Geometry check sheet. Reference: the model listing, model coordinates, mm. Give positions to 0.01 mm unless a question says otherwise; leave off trailing zeros. Write each loop counter-clockwise with the first axis right and the second up, starting at its lowest first coordinate (ties: lowest second). Pieces come first, ordered by that corner, then holes. Notation, with made-up numbers: M 21.25,61.25 L 58.25,61.25 A26 cw 58.25,94.25 Z; hole C 83,-15.5 d4. An arc over 180 degrees is marked long. Use one line per item in the form item = value. Start each with the question number.
Autodesk Inventor part; units mm, degrees
ref_plane "工作平面1" through (10, 22, 0) normal (-0.4333, -0.6373, -0.6373) x (0.8269, 0, -0.5623)
ref_plane "YZ Plane" through (0, 0, 0) normal (1, 0, 0) x (0, 1, 0)
ref_plane "XZ Plane" through (0, 0, 0) normal (0, 1, 0) x (-1, 0, 0)
sketch "草圖1" plane through (0, 0, 0) normal (0, 1, 0) x (-1, 0, 0)
  line L0 (0, 0) -> (-60, 0)
  line L1 (-60, 0) -> (-60, -44)
  line L2 (-60, -44) -> (0, -44)
  line L3 (0, -44) -> (0, 0)
  dimension "d0" = 60
  dimension "d1" = 44
extrude "擠出1" add sketch "草圖1" along normal mid plane 44
sketch "草圖2" plane through (0, 22, 0) normal (0, 1, 0) x (1, 0, 0)
  line L0 (0, 0) -> (60, 0)
  line L1 (10, 0) -> (60, 14)
  line L2 (60, 0) -> (60, 44)
  dimension "d4" = 10
  dimension "d5" = 30
extrude "擠出2" cut sketch "草圖2" against normal blind 60
sketch "草圖3" plane through (60, -22, -44) normal (1, 0, 0) x (0, 0, -1)
  line L0 (-30, 24) -> (-10, 44)
  line L1 (0, 44) -> (-44, 44)
  line L2 (-30, 44) -> (-30, 0)
  point P0 (-44, 22)
  point P1 (-30, 2)
  dimension "d8" = 20
  dimension "d9" = 20
ref_plane "工作平面1" through (10, 22, 0) normal (-0.4333, -0.6373, -0.6373) x (0.8269, 0, -0.5623)
sketch "草圖4" plane through (10, 22, 0) normal (-0.4333, -0.6373, -0.6373) x (0.8269, 0, -0.5623)
  line L0 (-15.1543, -12.3218) -> (93.717, -12.3218)
  line L1 (93.717, -12.3218) -> (93.717, 28.8166)
  line L2 (93.717, 28.8166) -> (-15.1543, 28.8166)
  line L3 (-15.1543, 28.8166) -> (-15.1543, -12.3218)
  point P0 (-8.2693, 13.3708)
extrude "擠出3" cut sketch "草圖4" against normal blind 40
mirror "鏡射1" about plane through (0, 0, 0) normal (0, 1, 0) of "擠出3"
properties part number "63"
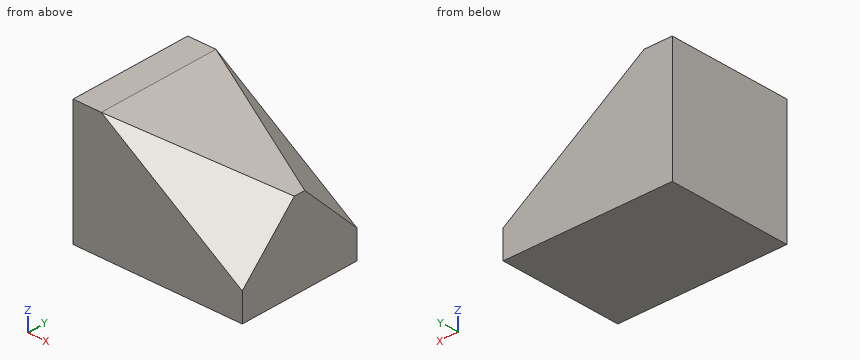
(1) Sectioned sample at B-B, the plane x = 22.5. Record the boundary of the cut face in (y, z), plus the area to 3 significant figures.
(2) Thickness scan on probe 1 along X at (y, z) = (-14.5, -10.5); probe 2 along Z at (x, y) = (40.5, 15.5); probe 3 along Z at (x, y) = (46.5, 2.5). Record the ranges inside material, lowest first. Write a range as [from, to].
(3) Sectioned sample at A-A, the plane z = -21. Record the boundary of the cut face in (x, y), plus the area to 3 significant figures.
(4) Depth check by flat-ended pin: pin 1 (1.5 mm diameter, centred on x = 39, y = 1, fed in from +Z); pin 2 (2 mm diameter, centred on y = -10.5, z = -18.5, fed in from +X); pin 3 (1 mm diameter, centred on x = 21.5, y = -1.5, fed in from +Z). Enter the tip coordinate at first touch or a pass-through.
Numbers:
q1.outline = M -22,-44 L 22,-44 L 22,-8.5 L 17,-3.5 L -17,-3.5 L -22,-8.5 Z
q1.area = 1,760 mm2
q2.probe_1 = [0, 36.47]
q2.probe_2 = [-44, -14.24]
q2.probe_3 = [-44, -10.22]
q3.outline = M 0,-22 L 40.88,-22 L 60,-9 L 60,9 L 40.88,22 L 0,22 Z
q3.area = 2,390 mm2
q4.pin_1 = -7.91
q4.pin_2 = 56.2
q4.pin_3 = -3.08
